Build history of the part. All positions in model axes, mm. Coordinates: 2 decimals unless noted, no trailing zeros. Order: outer loops, then holes, each group sorted by start corner. A loop starts at its lowest first (then second) coordinate and runs counter-clockwise, first axis right, second up. Notation, with made-up numbers: (70.5, -3.5) - (97.5, -3.5) arc R16 ccw to (97.5, 8.5) - close; hole circle Ø3 at (86.5, 5.25). An arc over 180 degrees is marked (long way). Write each question's results on one line, items separated by ' | '. Start each with the question number.
from build123d import *

# Parameters (mm, degrees)
SZKIC1_R                    = 8.6
DODANIE_WYCI_GNI_CIE1_DEPTH = 1.73
WYTNIJ_WYCI_GNI_CIE1_DEPTH  = 1.73


with BuildPart() as part:
    # Szkic1 → Dodanie-wyciągnięcie1 (new body)
    with BuildSketch(Plane.XY):
        Circle(SZKIC1_R)
    extrude(amount=DODANIE_WYCI_GNI_CIE1_DEPTH)

    # Szkic2 → Wytnij-wyciągnięcie1 (cut)
    with BuildSketch(Plane.XY.offset(1.73)):
        with BuildLine():
            Line((-2.583990936, 4.832534619), (-3.410143133, 5.969635568))
            ThreePointArc((-3.410143133, 5.969635568), (-4.04102361, 5.561991836), (-4.623668625, 5.087957689))
            Line((-4.623668625, 5.087957689), (-3.797516427, 3.950856741))
            ThreePointArc((-3.797516427, 3.950856741), (-4.433413129, 3.221063183), (-4.930985161, 2.390770869))
            Line((-4.930985161, 2.390770869), (-6.267727496, 2.825104782))
            ThreePointArc((-6.267727496, 2.825104782), (-6.53851355, 2.124491836), (-6.731252988, 1.398520008))
            Line((-6.731252988, 1.398520008), (-5.394510652, 0.964186094))
            ThreePointArc((-5.394510652, 0.964186094), (-5.48, 0), (-5.394510652, -0.964186094))
            Line((-5.394510652, -0.964186094), (-6.731252988, -1.398520008))
            ThreePointArc((-6.731252988, -1.398520008), (-6.53851355, -2.124491836), (-6.267727496, -2.825104782))
            Line((-6.267727496, -2.825104782), (-4.930985161, -2.390770869))
            ThreePointArc((-4.930985161, -2.390770869), (-4.433413129, -3.221063183), (-3.797516427, -3.950856741))
            Line((-3.797516427, -3.950856741), (-4.623668625, -5.087957689))
            ThreePointArc((-4.623668625, -5.087957689), (-4.04102361, -5.561991836), (-3.410143133, -5.969635568))
            Line((-3.410143133, -5.969635568), (-2.583990936, -4.832534619))
            ThreePointArc((-2.583990936, -4.832534619), (-1.693413129, -5.211789709), (-0.75, -5.428434397))
            Line((-0.75, -5.428434397), (-0.75, -6.833968466))
            ThreePointArc((-0.75, -6.833968466), (0, -6.875), (0.75, -6.833968466))
            Line((0.75, -6.833968466), (0.75, -5.428434397))
            ThreePointArc((0.75, -5.428434397), (1.693413129, -5.211789709), (2.583990936, -4.832534619))
            Line((2.583990936, -4.832534619), (3.410143133, -5.969635568))
            ThreePointArc((3.410143133, -5.969635568), (4.04102361, -5.561991836), (4.623668625, -5.087957689))
            Line((4.623668625, -5.087957689), (3.797516427, -3.950856741))
            ThreePointArc((3.797516427, -3.950856741), (4.433413129, -3.221063183), (4.930985161, -2.390770869))
            Line((4.930985161, -2.390770869), (6.267727496, -2.825104782))
            ThreePointArc((6.267727496, -2.825104782), (6.53851355, -2.124491836), (6.731252988, -1.398520008))
            Line((6.731252988, -1.398520008), (5.394510652, -0.964186094))
            ThreePointArc((5.394510652, -0.964186094), (5.48, 0), (5.394510652, 0.964186094))
            Line((5.394510652, 0.964186094), (6.731252988, 1.398520008))
            ThreePointArc((6.731252988, 1.398520008), (6.53851355, 2.124491836), (6.267727496, 2.825104782))
            Line((6.267727496, 2.825104782), (4.930985161, 2.390770869))
            ThreePointArc((4.930985161, 2.390770869), (4.433413129, 3.221063183), (3.797516427, 3.950856741))
            Line((3.797516427, 3.950856741), (4.623668625, 5.087957689))
            ThreePointArc((4.623668625, 5.087957689), (4.04102361, 5.561991836), (3.410143133, 5.969635568))
            Line((3.410143133, 5.969635568), (2.583990936, 4.832534619))
            ThreePointArc((2.583990936, 4.832534619), (1.693413129, 5.211789709), (0.75, 5.428434397))
            Line((0.75, 5.428434397), (0.75, 6.833968466))
            ThreePointArc((0.75, 6.833968466), (0, 6.875), (-0.75, 6.833968466))
            Line((-0.75, 6.833968466), (-0.75, 5.428434397))
            ThreePointArc((-0.75, 5.428434397), (-1.693413129, 5.211789709), (-2.583990936, 4.832534619))
        make_face()
    extrude(amount=-WYTNIJ_WYCI_GNI_CIE1_DEPTH, mode=Mode.SUBTRACT)


solid = part.part
Item 1: Flat gauge pin, fed straight in: P1, Ø3, axis at x = 3, y = -1, coming from the -Z side. Where does the tip first touch, or does it go through?
Item 2: Pull direction Y, two halves, no side cores. Call faces 1 (the cylindrical face through (4.44, 3.21, 0.88)), 2 (the cylindrical face through (-8.59, 0.38, 0.85)), 3 (the flat face through (0.75, 6, 1)): released by +Y, released by -Y, zero draft, split by the parting line, or undercut.
Item 3: Slice it at C-C (x = 4). Write the cut outline in (y, z), then the cut area to 3 significant figures.
Item 4: Slice it at A-A (y = 0). Write the cut outline in (x, z).
Item 5: Slice it at B-B (x = 0). Write the cut outline in (y, z) (3 decimals), then the cut area to 3 significant figures.
Item 6: Probe probe 1 along X at (y, z) = (5.5, 1.2) (3 decimals); probe 2 along X at (y, z) = (-5, 0.55); probe 3 along Y at (x, z) = (-7.25, 0.5). List the from-to ranges inside material, lowest first.
Item 7: Slice it at D-D (x = -5.75). Write the cut outline in (y, z), then the cut area to 3 significant figures.
Resolved:
1) P1: through
2) face 1: undercut | face 2: split by the parting line | face 3: undercut
3) outline: (-7.61, 0) - (-5.59, 0) - (-5.59, 1.73) - (-7.61, 1.73) - close; (-4.23, 0) - (-3.75, 0) - (-3.75, 1.73) - (-4.23, 1.73) - close; (3.75, 0) - (4.23, 0) - (4.23, 1.73) - (3.75, 1.73) - close; (5.59, 0) - (7.61, 0) - (7.61, 1.73) - (5.59, 1.73) - close | area: 8.67 mm^2
4) outline: (-8.6, 0) - (-5.48, 0) - (-5.48, 1.73) - (-8.6, 1.73) - close; (5.48, 0) - (8.6, 0) - (8.6, 1.73) - (5.48, 1.73) - close
5) outline: (-8.6, 0) - (-6.875, 0) - (-6.875, 1.73) - (-8.6, 1.73) - close; (6.875, 0) - (8.6, 0) - (8.6, 1.73) - (6.875, 1.73) - close | area: 5.97 mm^2
6) probe 1: -6.611 to -4.125, -3.069 to -0.75, 0.75 to 3.069, 4.125 to 6.611 | probe 2: -7 to -4.56, -2.71 to -2.24, 2.24 to 2.71, 4.56 to 7 | probe 3: -4.63 to 4.63
7) outline: (-6.4, 0) - (-2.66, 0) - (-2.66, 1.73) - (-6.4, 1.73) - close; (-1.08, 0) - (1.08, 0) - (1.08, 1.73) - (-1.08, 1.73) - close; (2.66, 0) - (6.4, 0) - (6.4, 1.73) - (2.66, 1.73) - close | area: 16.7 mm^2
